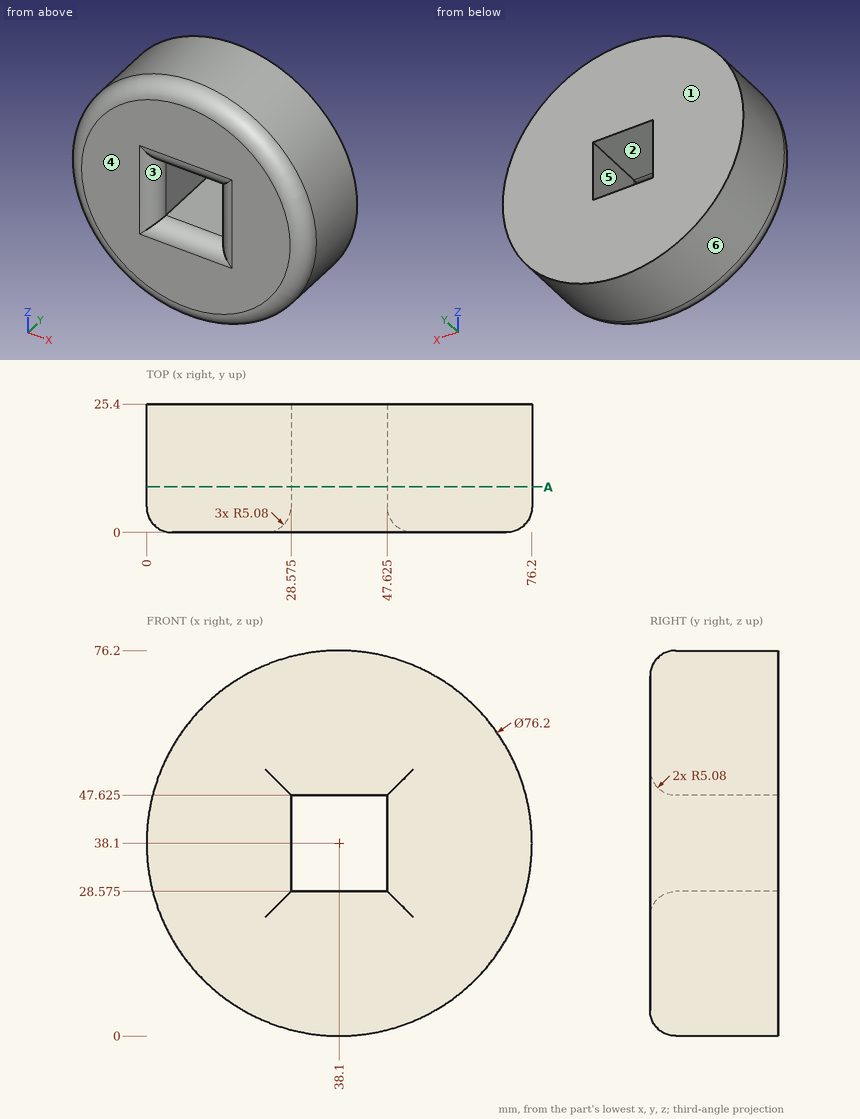
Geometry check sheet. Reference: drawing and pictorial views, mm from the part's lowest x, y, z. A direction names the side the tool comes from. Coordinates: 2 decimals unless noted, no trailing zeros. Write each loop counter-clockwise with the first axis right and the second up, starting at its lowest first coordinate (ties: lowest second). Pieces come first, ordered by that corner, then holes. Notation, with made-up numbers: (23.5, 11) - (60.5, 11) arc R22 ccw to (60.5, 42) - close; hole circle Ø7 at (29, 85). An arc over 180 degrees is marked (long way). One line per question, with ' | ' between items. Start each with the question number.
1. Section check A-A (y = 9). Enter the section's corners in (x, z) (3 decimals), plus the area to 3 significant figures.
2. Material ranges on line 1 along X through (y, z) = (11, 34.5) (3 decimals); line 2 along X through (y, z) = (8.25, 47) (3 decimals); line 3 along Z through (x, y) = (35.5, 16) (3 decimals), recorded low to high.
3. Draft check along Z on the marked faces 4, 5 and 6. Enter one of: released by +Z, released by -Z, zero draft, split by the parting line, or undercut.
4. Gauge pin test, flat ends, axial feed: P1, Ø9.5, axis at x = 41.5, y = 10.5, coming from the -Z side; P2, Ø9.5, axis at x = 37, y = 19.5, coming from the +Z side; P3, Ø3, axis at y = 15, z = 28, coming from the +X side. Record the tip position at first contact, or that the pin passes through.
5. Access from +Z, -Z, +X, -X, +Y, -Y to the whole of each face (thin tool, end or side, straight path). Record for the marked faces 1, 2 and 3.
Computed values:
1) outline: circle Ø76.2 at (38.1, 38.1); hole (28.575, 28.575) - (47.625, 28.575) - (47.625, 47.625) - (28.575, 47.625) - close | area: 4,200 mm²
2) line 1: 0.17 to 28.575, 47.625 to 76.03 | line 2: 1.054 to 28.575, 47.625 to 75.146 | line 3: 0.089 to 28.575, 47.625 to 76.111
3) face 4: zero draft | face 5: undercut | face 6: split by the parting line
4) P1: z = 0 | P2: z = 76.2 | P3: x = 75.22
5) face 1: +Z, -Z, +X, -X, +Y | face 2: +Y, -Y | face 3: -Y
